from build123d import *

# Parameters (mm, degrees)
FILLET1_R = 3
FILLET2_R = 3


with BuildPart() as part:
    # Sketch1 → Revolve1 (revolve)
    with BuildSketch(Plane.XY, mode=Mode.PRIVATE) as revolve1_sk:
        Polygon((15, 31.5), (15, 37.5), (0, 37.5), (0, 25), (6, 25), (6, 31.5), align=None)
    revolve(revolve1_sk.sketch.rotate(Axis((0, 0, 0), (1, 0, 0)), 90), axis=Axis((0, 0, 0), (1, 0, 0)))

    # Fillet1
    fillet1_edges = [part.edges().sort_by_distance(p)[0] for p in [
        (15, 0, -37.5),
        (15, 0, -31.5),
    ]]
    fillet(fillet1_edges, radius=FILLET1_R - 0.0001)  # a hair under: the kernel refuses the full size

    # Fillet2
    fillet2_edges = [part.edges().sort_by_distance(p)[0] for p in [
        (6, 0, -31.5),
        (0, 0, -37.5),
    ]]
    fillet(fillet2_edges, radius=FILLET2_R)


solid = part.part
Could you check a few things on this model? Use its own coordinates, in mm. A direction names the side the tool comes from. Coordinates: 2 decimals unless noted, no trailing zeros. Write each loop counter-clockwise with the first axis right and the second up, starting at its lowest first coordinate (ties: lowest second). Pieces come first, ordered by that corner, then holes. Notation, with made-up numbers: (47.5, 57.25) - (57.5, 57.25) arc R27 ccw to (57.5, 87.25) - close; hole circle Ø11 at (10.25, -40). An arc over 180 degrees is marked (long way). Put each result on its own line as item: value. Start each with the question number.
Q1. I want a section at D-D on x = 13.5. Write out the boundary of the cut face in (y, z).
Q2. I want a section at C-C on x = 7.25. Write out the boundary of the cut face in (y, z), plus the area to 3 significant figures.
Q3. I'm going to push flat-ended pins straight in: P1, Ø2, axis at x = 11.5, y = -6, coming from the -Z side; P2, Ø1, axis at x = 11, z = -8.5, coming from the +Y side; P3, Ø2, axis at x = 10.5, y = -26, coming from the +Z side. Where does each tip first touch, or does it pass through?
Q4. Thinking about a two-plate mould opening in Y: for faces 3 (the cylindrical face through (7.44, 33.27, 17.3)), 4 (the flat face through (6, 25.2, 0.1)), 5 (the flat face through (0, -18, 18)), which applies, pulls with the +Y half, pulls with the -Y half, needs draft (parallel to the pull), parting line crosses it, or undercut?
Q5. Please list where these lines run through material, in increasing order: L1, parallel to Y at x = 10.85, z = 0; L2, parallel to X at y = 26, z = -10.5; L3, parallel to Y at x = 9, z = -22.5.
Q6. Which directions (+Z, -Z, +X, -X, +Y, -Y) give clear straight access to the entire face, cutting with the end or side of a thin tool? Please do faces 1 (the cylindrical face through (10.521, -31.232, -4.101)), 2 (the cylindrical face through (3.042, -7.509, 23.846)).
Checks:
1. outline: circle Ø74.2 at (0, 0); hole circle Ø63.8 at (0, 0)
2. outline: circle Ø75 at (0, 0); hole circle Ø61.87 at (0, 0)
2. area: 1,410 mm²
3. P1: z = -37.17
3. P2: y = 36.64
3. P3: z = 27.95
4. face 3: parting line crosses it
4. face 4: undercut
4. face 5: needs draft
5. L1: -37.5 to -31.5, 31.5 to 37.5
5. L2: 0 to 6
5. L3: -30 to -22.05, 22.05 to 30
6. face 1: +X
6. face 2: +X, -X
